```python
from build123d import *

# Parameters (mm, degrees)
F3_R     = 5.08
F4_DEPTH = 3.175


with BuildPart() as f1:
    # F0 (on Front) → F1 (revolve)
    with BuildSketch(Plane.XZ):
        with BuildLine():
            ThreePointArc((12.3825, 1.23411), (11.259968, 0.769142), (10.795, -0.35339))
            Line((10.795, -0.35339), (10.795, -7.33839))
            ThreePointArc((10.795, -7.33839), (11.259968, -8.460922), (12.3825, -8.92589))
            ThreePointArc((12.3825, -8.92589), (13.505032, -8.460922), (13.97, -7.33839))
            Line((13.97, -7.33839), (13.97, -0.35339))
            ThreePointArc((13.97, -0.35339), (13.505032, 0.769142), (12.3825, 1.23411))
        make_face()
    revolve(axis=Axis((0, 0, 14.801255), (0, 0, 1)))

    # F3 (on offset) → F4 (join)
    with BuildSketch(Plane.XZ.offset(10.795)):
        with Locations((0, -3.84589)):
            Circle(F3_R)
    extrude(amount=F4_DEPTH)

    # F0 (on Front) → F5 (revolve, cut)
    with BuildSketch(Plane.XZ):
        with BuildLine():
            Line((10.795, -7.33839), (10.795, -0.35339))
            ThreePointArc((10.795, -0.35339), (11.259968, 0.769142), (12.3825, 1.23411))
            Line((12.3825, 1.23411), (7.964968, 1.23411))
            Line((7.964968, 1.23411), (7.964968, -8.92589))
            Line((7.964968, -8.92589), (12.3825, -8.92589))
            ThreePointArc((12.3825, -8.92589), (11.259968, -8.460922), (10.795, -7.33839))
        make_face()
    revolve(axis=Axis((0, 0, 14.801255), (0, 0, 1)), mode=Mode.SUBTRACT)


solid = f1.part
```
Model file for the job. Use its own axes, mm. Coordinates: 2 decimals unless noted, no trailing zeros. Order: outer loops, then holes, each group sorted by start corner. A loop starts at its lowest first (then second) coordinate and runs counter-clockwise, first axis right, second up. Notation, with made-up numbers: (31, -30) -> (89, -30) arc R19 ccw to (89, -7) -> close; hole circle Ø4 at (18.5, 55). An arc over 180 degrees is marked (long way). Answer as a JSON object with one key per item and string values. Group by question number.
1) Flat gauge pin, fed straight in: pin 1 (5 mm diameter, centred on x = -7, y = -5.5, fed in from +Z). Where does the tip first touch, or does it go through?
2) Pull direction Y, two halves, no side cores. Call faces 1 (the face through (0, -13.97, -4)), 2 (the face through (0.56, 13.96, -3.8)), 3 (the face through (-7.956, 7.296, -3.895)): +Y half, -Y half, draft (parallel to the pull), parting line (faces both ways), or undercut.
3) Cut at B-B, the plane z = -6.5. Write the cut outline in (x, y) (3 decimals).
4) Cut at A-A, the plane z = -5. Write the cut outline in (x, y) (3 decimals), then the cut area to 3 significant figures.
5) Drill centre lines: L1, parallel to X at y = 0, z = -2 (3 decimals); L2, parallel to X at y = -5.25, z = -4. Where is each one in solid material? Low to high.
Check values:
{
 "1": {"pin 1": "stops at z = 0.9"},
 "2": {"face 1": "-Y half", "face 2": "parting line", "face 3": "undercut"},
 "3": {"outline": "(-4.332, -13.97) -> (4.332, -13.97) -> (4.332, -13.282) arc R13.97 ccw (long way) to (-4.332, -13.282) -> close; hole circle Ø21.59 at (0, 0)"},
 "4": {"outline": "(-4.947, -13.97) -> (4.947, -13.97) -> (4.947, -13.065) arc R13.97 ccw (long way) to (-4.947, -13.065) -> close; hole circle Ø21.59 at (0, 0)", "area": "250 mm²"},
 "5": {"L1": "x = -13.97 to -10.795, 10.795 to 13.97", "L2": "x = -12.95 to -9.43, 9.43 to 12.95"}
}
